Source: three-view drawing plus pictorial views. Frame: mm from the lowest corner of the part. A direction names the side the tool comes from. Coordinates: 2 decimals unless noted, no trailing zeros. Order: outer loops, then holes, each group sorted by start corner. A loop starts at its lowest first (then second) coordinate and runs counter-clockwise, first axis right, second up. Notation, with made-up numbers: M 77.5,55 L 107.5,55 A21 ccw 107.5,65 Z; hole C 79,26 d8. An arc over 180 degrees is marked long. One line per question, with ' | ' between items.
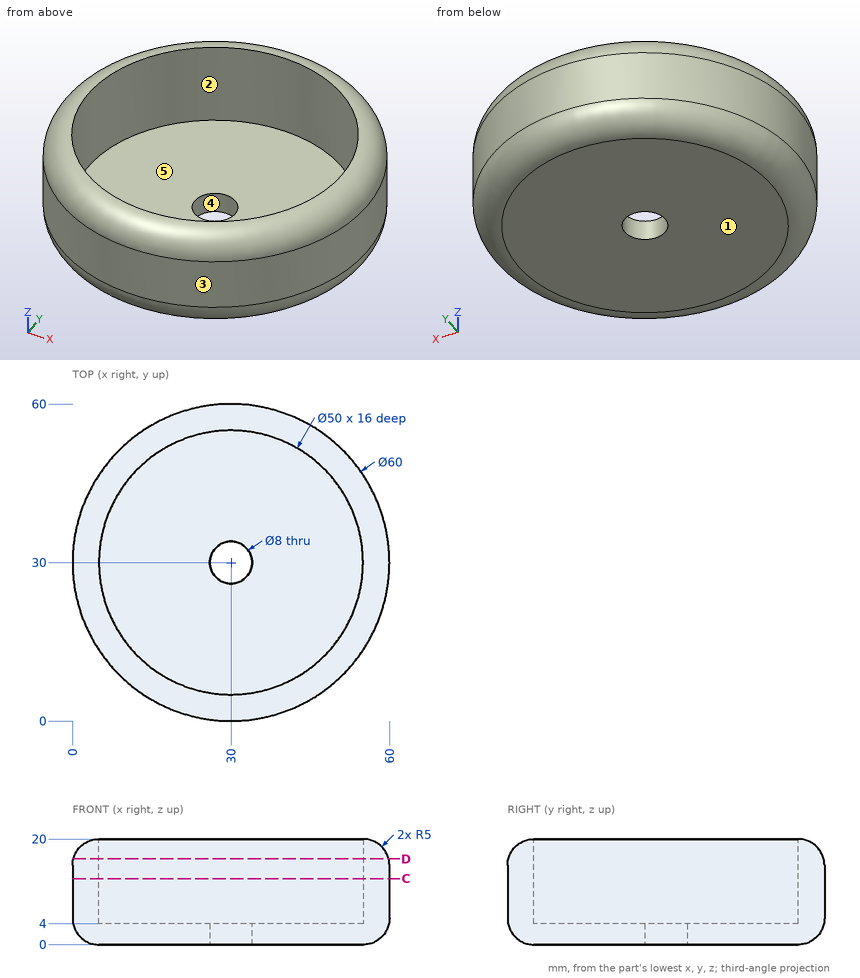
1. Material intervals for line 1 (Y direction, x = 30, z = 11); line 2 (Z direction, x = 44, y = 31.5); line 3 (Y direction, x = 37, z = 16.25), sorted ascending. Write a range as [from, to].
Response values:
line 1: y = [0, 5], [55, 60] | line 2: z = [0, 4] | line 3: y = [0.99, 6], [54, 59.01]
2. Section D-D, the plane z = 16.25. Output: boundary loops of the cut face in (x, y).
Response values:
outline: C 30,30 d59.68; hole C 30,30 d50
3. Section C-C, the plane z = 12.5. Output: boundary loops of the cut face in (x, y), and give its area (3 significant figures).
Response values:
outline: C 30,30 d60; hole C 30,30 d50 | area: 864 mm^2
4. Pin query (flat end, axial travel): P1, Ø8, axis at x = 20, z = 7, coming from the -Y side; P2, Ø3, axis at x = 48.5, z = 4, coming from the -Y side; P3, Ø2, axis at y = 21, z = 6, coming from the +X side; P4, Ø7, axis at x = 30, y = 30, coming from the +Z side. Return the tip coordinate at first contact, or that it passes through.
Response values:
P1: stops at y = 0.61 | P2: stops at y = 5.36 | P3: stops at x = 58.91 | P4: passes through
5. Access query for the marked faces 4 and 5. Directions: +Z, -Z, +X, -X, +Y, -Y. A direction counts if a zero-diameter tool reaches every point of the face in a straight line with its end or side. Return the directions, or none.
Response values:
face 4: +Z, -Z | face 5: +Z
6. Draft query along Y for the marked faces 1, 2 and 3. Return one class per face: pulls with the +Y half, pulls with the -Y half, needs draft (parallel to the pull), parting line crosses it, or undercut.
Response values:
face 1: needs draft | face 2: undercut | face 3: parting line crosses it
